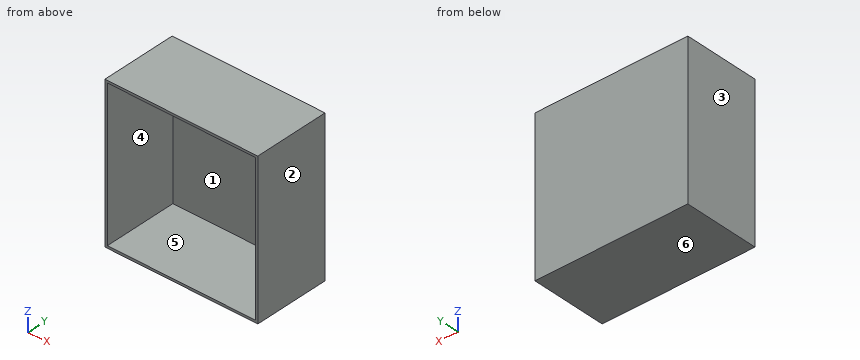
from build123d import *

# Parameters (mm, degrees)
SKETCH1_W           = 203.2
SKETCH1_H           = 203.2
BOSS_EXTRUDE1_DEPTH = 2.54
SKETCH2_W           = 203.2
SKETCH2_H           = 203.2
SKETCH2_W_2         = 196.85
SKETCH2_H_2         = 196.85
BOSS_EXTRUDE2_DEPTH = 98.425


with BuildPart() as part:
    # Sketch1 → Boss-Extrude1 (new body)
    with BuildSketch(Plane(origin=(0, 0, 0), x_dir=(1, 0, 0), z_dir=(0, 1, 0))):
        with Locations((101.6, -101.6)):
            Rectangle(SKETCH1_W, SKETCH1_H)
    extrude(amount=BOSS_EXTRUDE1_DEPTH)

    # Sketch2 → Boss-Extrude2 (add)
    with BuildSketch(Plane.XZ):
        with Locations((101.6, 101.6)):
            Rectangle(SKETCH2_W, SKETCH2_H)
        with Locations((101.6, 101.6)):
            Rectangle(SKETCH2_W_2, SKETCH2_H_2, mode=Mode.SUBTRACT)
    extrude(amount=BOSS_EXTRUDE2_DEPTH)


solid = part.part
Could you check a few things on this model? Use its own coordinates, in mm. Face numbers are marked on the shaded views. A direction names the side the tool comes from. Coordinates: 2 decimals unless noted, no trailing zeros. Write each loop counter-clockwise with the first axis right and the second up, starting at its lowest first coordinate (ties: lowest second). Pieces come first, ordered by that corner, then holes. Notation, with made-up numbers: M -33.75,-26 L -2.75,-26 A17 cw -2.75,-16 Z; hole C -4.75,-20 d11. An arc over 180 degrees is marked long. One line per question, with ' | ' between items.
1) Imagine slicing it at C-C, the plane z = 53.5. Write out the boundary of the cut face in (x, y) (3 decimals).
Checks:
outline: M 0,-98.425 L 3.175,-98.425 L 3.175,0 L 200.025,0 L 200.025,-98.425 L 203.2,-98.425 L 203.2,2.54 L 0,2.54 Z
2) If we mould it in two halves opening along X, with no side actions, what happens to the marked faces 3, 4, 5 and 6? For each: released by +X, released by -X, zero draft, split by the parting line, or undercut.
Checks:
face 3: released by -X | face 4: undercut | face 5: undercut | face 6: zero draft
3) Imagine slicing it at A-A, the plane y = -89. Write out the boundary of the cut face in (x, z) (3 decimals).
Checks:
outline: M 0,0 L 203.2,0 L 203.2,203.2 L 0,203.2 Z; hole M 3.175,3.175 L 200.025,3.175 L 200.025,200.025 L 3.175,200.025 Z
4) Imagine slicing it at B-B, the plane x = 25. Write out the boundary of the cut face in (y, z) (3 decimals).
Checks:
outline: M -98.425,0 L 2.54,0 L 2.54,203.2 L -98.425,203.2 L -98.425,200.025 L 0,200.025 L 0,3.175 L -98.425,3.175 Z
5) For the marked faces 1 and 2, which set-ups out of +Z, -Z, +X, -X, +Y, -Y let a thin tool reach every point of the face, with its end or its side?
Checks:
face 1: -Y | face 2: +Z, -Z, +X, +Y, -Y
6) I need wall thicknesses on probe 1 along Z at (x, y) = (15, -16) (3 decimals); probe 2 along Y at (x, z) = (124.5, 147). Which ranges of each line are inside material? Lowest first, please. Write a range as [from, to].
Checks:
probe 1: [0, 3.175], [200.025, 203.2] | probe 2: [0, 2.54]
7) For pin 1 Ø5 at (x, z) = (113.5, 82) entering from -Y; pin 2 Ø4 at (y, z) = (-25, 36) entering from -X, each with a flat end and sliding along its axis, tell me the tip position at first contact or that it passes through.
Checks:
pin 1: y = 0 | pin 2: x = 0
